Could you check a few things on this model? Use its own coordinates, in mm. A direction names the side the tool comes from. Round coordinates to 2 decimals unless told otherwise and drop trailing zeros. Order: outer loops, then holes, each group sorted by start corner. A loop starts at its lowest first (then second) coordinate and runs counter-clockwise, first axis right, second up. Notation, with made-up numbers: M -32.75,-36 L -11.75,-36 A25 cw -11.75,-9 Z; hole C 15,57 d11. An arc over 180 degrees is marked long. Write each question's results on one line, items separated by ' | '. Start each with the question number.
1. Suppose I cut it at B-B on x = -12.7. Write out the boundary of the cut face in (y, z).
2. For faces 5 (the cylindrical face through (-0.586, 3.815, -12.522)), 6 (the flat face through (-3.8, 0, 0)), which set-ups out of +Z, -Z, +X, -X, +Y, -Y let a thin tool reach every point of the face, with its end or its side?
3. I'm going to push flat-ended pins straight in: pin 1 (3 mm diameter, centred on x = -26, z = 13, fed in from -Y); pin 2 (8 mm diameter, centred on x = -17, z = 26, fed in from +Y); pin 3 (10 mm diameter, centred on x = 18, z = 17, fed in from -Y); pin 4 (3 mm diameter, centred on x = -1, y = 25.5, fed in from +Z). Where does each tip first touch, or does it pass through?
4. Please list where these lines run through material, in increasing order: L1, parallel to X at y = 39.5, z = 58.5; L2, parallel to Y at x = -20, z = 20; L3, parallel to Y at x = -17.5, z = 55.5.
5. Suppose I cut it at C-C on z = 19.5. Write out the boundary of the cut face in (x, y), and give its area (3 significant figures).
6. Suppose I cut it at A-A on y = 0. Write out the boundary of the cut face in (x, z).
7. We'd pull the mould along X, two halves only. Please class faces 1 (the flat face through (-15, 9, -25.4)), 2 (the cylindrical face through (-4.4, 2.67, -12.52)), 3 (the conical face through (-17.13, -19.97, 17.94)), 4 (the conical face through (11, -45, 66)): released by +X, released by -X, zero draft, split by the parting line, or undercut.
8. Suppose I cut it at D-D on z = 3.5. Write out the boundary of the cut face in (x, y), and give its area (3 significant figures).
from build123d import *

# Parameters (mm, degrees)
F2_R     = 7.582506
F3_DEPTH = 25.4
F4_R     = 8.897852
F5_DEPTH = 25.4


with BuildPart() as f1:
    # F0 (on Front) → F1 (revolve)
    with BuildSketch(Plane.XZ):
        Polygon((0, -25.4), (0, 0), (40.193673, 64.737228), (37.751768, 66.253343), (-3.383222, 0), (-12.7, 0), (-12.7, -25.4), align=None)
    revolve(axis=Axis((-12.7, 0, -12.7), (0, 0, 1)))

    # F2 (on face) → F3 (cut)
    with BuildSketch(Plane.XY):
        with Locations((-12.7, 0)):
            Circle(F2_R)
    extrude(amount=-F3_DEPTH, mode=Mode.SUBTRACT)

    # F4 (on Top) → F5 (cut)
    with BuildSketch(Plane.XY):
        with Locations((-12.889439, 0)):
            Circle(F4_R)
    extrude(amount=-F5_DEPTH, mode=Mode.SUBTRACT)


solid = f1.part
Filled sheet:
1) outline: M -52.89,64.74 L -12.7,0 L -12.7,-25.4 L -8.9,-25.4 L -8.9,0 L -9.32,0 L -50.45,66.25 Z; M 8.9,-25.4 L 12.7,-25.4 L 12.7,0 L 52.89,64.74 L 50.45,66.25 L 9.32,0 L 8.9,0 Z
2) face 5: -Z | face 6: +Z
3) pin 1: stops at y = -17.59 | pin 2: stops at y = 31.08 | pin 3: passes through | pin 4: stops at z = 32.6
4) L1: x = -41.73 to -35.56, 10.16 to 16.33 | L2: y = -24.03 to -20.47, 20.47 to 24.03 | L3: y = -46.91 to -43.51, 43.51 to 46.91
5) outline: C -12.7,0 d49.61; hole C -12.7,0 d42.85 | area: 491 mm^2
6) outline: M -65.59,64.74 L -25.4,0 L -25.4,-25.4 L -21.79,-25.4 L -21.79,0 L -22.02,0 L -63.15,66.25 Z; M -3.99,-25.4 L 0,-25.4 L 0,0 L 40.19,64.74 L 37.75,66.25 L -3.38,0 L -3.99,0 Z
7) face 1: zero draft | face 2: undercut | face 3: undercut | face 4: split by the parting line
8) outline: C -12.7,0 d29.75; hole C -12.7,0 d22.98 | area: 280 mm^2
